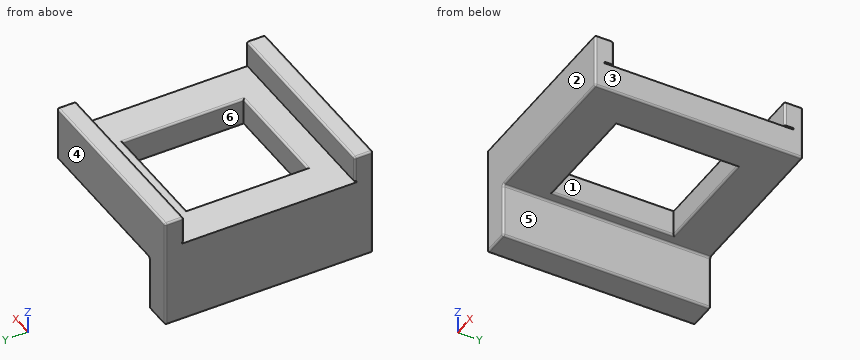
from build123d import *

# Parameters (mm, degrees)
BOX_W            = 1
BOX_H            = 4
BOX_DEPTH        = 3
BOX001_W         = 1
BOX001_H         = 4
BOX001_DEPTH     = 3
SKETCH003_W      = 60
SKETCH003_H      = 65
EXTRUDE003_DEPTH = 15
EXTRUDE001_DEPTH = 51
SKETCH_W         = 102
SKETCH_H         = 102
EXTRUDE_DEPTH    = 15
SKETCH002_W      = 15
SKETCH002_H      = 30
EXTRUDE002_DEPTH = 56
FILLET_R         = 1
FILLET001_R      = 1


with BuildPart() as cube:
    # Box → Box (new body)
    with BuildSketch(Plane(origin=(-51, 47, 14.7), x_dir=(1, 0, 0), z_dir=(0, 0, 1))):
        with Locations((0.5, 2)):
            Rectangle(BOX_W, BOX_H)
    extrude(amount=BOX_DEPTH)


with BuildPart() as cube001:
    # Box001 → Box001 (new body)
    with BuildSketch(Plane(origin=(-51, -51, 14.7), x_dir=(1, 0, 0), z_dir=(0, 0, 1))):
        with Locations((0.5, 2)):
            Rectangle(BOX001_W, BOX001_H)
    extrude(amount=BOX001_DEPTH)


with BuildPart() as extrude003:
    # Sketch003 (on Face42 of Fillet) → Extrude003 (new body)
    with BuildSketch(Plane.XY.offset(15)):
        Rectangle(SKETCH003_W, SKETCH003_H)
    extrude(amount=-EXTRUDE003_DEPTH)


with BuildPart() as extrude001:
    # Sketch001 (on Sketch) → Extrude001 (new body, symmetric)
    with BuildSketch(Plane.YZ):
        Polygon((-56, 0), (-56, 30), (-46, 30), (-46, 15.9), (-51, 15.9), (-51, 15), (-46, 15), (-46, 0), align=None)
        Polygon((56, 0), (56, 30), (46, 30), (46, 15.9), (51, 15.9), (51, 15), (46, 15), (46, 0), align=None)
    extrude(amount=EXTRUDE001_DEPTH, both=True)


with BuildPart() as fusion:
    # Sketch → Extrude (new body)
    with BuildSketch(Plane.XY):
        Rectangle(SKETCH_W, SKETCH_H)
    extrude(amount=EXTRUDE_DEPTH)

    # Fusion: union Extrude001
    add(extrude001.part)


with BuildPart() as fusion002:
    # Sketch002 → Extrude002 (new body, symmetric)
    with BuildSketch(Plane.XZ):
        with Locations((-43.5, -15)):
            Rectangle(SKETCH002_W, SKETCH002_H)
    extrude(amount=EXTRUDE002_DEPTH, both=True)

    # Fusion001: union Fusion
    add(fusion.part)

    # Fillet
    fillet_edges = [fusion002.edges().sort_by_distance(p)[0] for p in [
        (-36, 0, 0),
        (-36, 0, -30),
        (-36, 56, -15),
        (-36, -56, -15),
        (-51, 0, -30),
        (-43.5, 56, -30),
        (-43.5, -56, -30),
        (51, 0, 0),
        (7.5, -56, 0),
        (7.5, 56, 0),
        (-51, 56, 0),
        (0, 56, 30),
        (51, 56, 15),
        (0, 46, 30),
        (51, 46, 22.95),
        (-51, 46, 22.95),
        (51, 51, 30),
        (-51, 51, 30),
        (51, -56, 15),
        (0, -56, 30),
        (-51, -56, 0),
        (0, -46, 30),
        (51, -51, 30),
        (-51, -51, 30),
        (51, -46, 22.95),
        (-51, -46, 22.95),
    ]]
    fillet(fillet_edges, radius=FILLET_R)

    # Cut: cut Extrude003
    add(extrude003.part, mode=Mode.SUBTRACT)

    # Fillet001
    fillet001_edges = [fusion002.edges().sort_by_distance(p)[0] for p in [
        (0, 32.5, 0),
        (30, 0, 0),
        (0, -32.5, 0),
        (-30, 0, 0),
        (0, 32.5, 15),
        (30, 0, 15),
        (0, -32.5, 15),
        (-30, 0, 15),
    ]]
    fillet(fillet001_edges, radius=FILLET001_R)

    # Fusion002: union Cube, Cube001
    add(cube.part)
    add(cube001.part)


solid = fusion002.part
Work out the finished part from the listing and answer in its coordinate system (mm). Face numbers are marked on the shaded views. A direction names the side the tool comes from. Round coordinates to 2 decimals unless told otherwise and drop trailing zeros. Write each loop counter-clockwise with the first axis right and the second up, starting at its lowest first coordinate (ties: lowest second). Pieces come first, ordered by that corner, then holes. Notation, with made-up numbers: M 9,-23 L 33,-23 A27 ccw 33,8 Z; hole C -37.75,67.5 d11. An arc over 180 degrees is marked long. Use a Markdown table: item, result.
1) The part is cut by section A-A on y = -12. Give the vertices of the cut face in (x, z).
Taken from the geometry:
| item | result |
|---|---|
| outline | M -51,-29 A1 ccw -50,-30 L -37,-30 A1 ccw -36,-29 L -36,-1 A1 cw -35,0 L -31,0 A1 ccw -30,1 L -30,14 A1 ccw -31,15 L -51,15 Z; M 30,1 A1 ccw 31,0 L 50,0 A1 ccw 51,1 L 51,15 L 31,15 A1 ccw 30,14 Z |
2) Which of the six approach directions +Z, -Z, +X, -X, +Y, -Y give full straight-line access (tool end or side, diameter ignored) to the marked faces 4, 5 and 6?
Taken from the geometry:
| item | result |
|---|---|
| face 4 | +Z, -Z, +X, -X, +Y |
| face 5 | -Z, +X, +Y, -Y |
| face 6 | +Z, -Z |
3) The part is cut by section B-B on x = 18.5. Give the vertices of the cut face in (y, z), plus the area to 3 significant figures.
Taken from the geometry:
| item | result |
|---|---|
| outline | M -56,1 A1 ccw -55,0 L -33.5,0 A1 ccw -32.5,1 L -32.5,14 A1 ccw -33.5,15 L -51,15 L -51,15.9 L -46,15.9 L -46,29 A1 ccw -47,30 L -55,30 A1 ccw -56,29 Z; M 32.5,1 A1 ccw 33.5,0 L 55,0 A1 ccw 56,1 L 56,29 A1 ccw 55,30 L 47,30 A1 ccw 46,29 L 46,15.9 L 51,15.9 L 51,15 L 33.5,15 A1 ccw 32.5,14 Z |
| area | 994 mm2 |
4) Flat-ended cylindrical pins translate along their axes: pin 1 (2 mm diameter, centred on x = 38, y = -20, fed in from -Z); pin 2 (0.5 mm diameter, centred on y = 49.5, z = 15.5, fed in from +X); pin 3 (2 mm diameter, centred on y = -38.5, z = -9.5, fed in from +X); pin 4 (12 mm diameter, centred on x = -20, y = 5, fed in from -Z). Find the tip coordinate at first contact, or state that the pin passes through.
Taken from the geometry:
| item | result |
|---|---|
| pin 1 | stops at z = 0 |
| pin 2 | stops at x = -50 |
| pin 3 | stops at x = -36 |
| pin 4 | passes through |
5) Determine the mould class of the marked faces 1, 2 and 3 for opening direction Y: pulls with the +Y half, pulls with the -Y half, needs draft (parallel to the pull), parting line crosses it, or undercut.
Taken from the geometry:
| item | result |
|---|---|
| face 1 | undercut |
| face 2 | pulls with the -Y half |
| face 3 | needs draft |
6) The part is cut by section C-C on z = 3. Give the vertices of the cut face in (x, y), plus the area to 3 significant figures.
Taken from the geometry:
| item | result |
|---|---|
| outline | M -51,-55 A1 ccw -50,-56 L 50,-56 A1 ccw 51,-55 L 51,55 A1 ccw 50,56 L -50,56 A1 ccw -51,55 Z; hole M -30,-32.5 L 30,-32.5 L 30,32.5 L -30,32.5 Z |
| area | 7,520 mm2 |
7) Consider line 1 (Y direction, x = 6.5, z = 12.5); line 2 (X direction, y = -10, z = 14); line 3 (Y direction, x = 10.5, z = 25.5). Determine where each line is inside the solid, lowest interval first. Write a range as [from, to].
Taken from the geometry:
| item | result |
|---|---|
| line 1 | y = [-56, -32.5], [32.5, 56] |
| line 2 | x = [-51, -30], [30, 51] |
| line 3 | y = [-56, -46], [46, 56] |
8) The part is cut by section D-D on z = 18. Give the vertices of the cut face in (x, y), plus the area to 3 significant figures.
Taken from the geometry:
| item | result |
|---|---|
| outline | M -51,-55 A1 ccw -50,-56 L 50,-56 A1 ccw 51,-55 L 51,-47 A1 ccw 50,-46 L -50,-46 A1 ccw -51,-47 Z; M -51,47 A1 ccw -50,46 L 50,46 A1 ccw 51,47 L 51,55 A1 ccw 50,56 L -50,56 A1 ccw -51,55 Z |
| area | 2,040 mm2 |
